CAD build for the part. Positions are in the model's coordinates, mm. A direction names the side the tool comes from. Round coordinates to 2 decimals unless told otherwise and drop trailing zeros. Write each loop counter-clockwise with the first axis right and the second up, starting at its lowest first coordinate (ties: lowest second). Pieces come first, ordered by that corner, then holes. Notation, with made-up numbers: (-11.5, 59.5) - (9.5, 59.5) arc R23 ccw to (9.5, 92.5) - close; hole circle Ø8 at (36, 61). An arc over 180 degrees is marked (long way). Use one line per item in the form item = value. Start each with the question number.
Item 1: Band-saw the part on B-B, the plane x = -9.5. List the corners of the cut face in (y, z).
Item 2: Band-saw the part on A-A, the plane z = -8.5. List the corners of the cut face in (x, y).
Item 3: Drill centre lines: L1, parallel to Y at x = 13, z = -8.25; L2, parallel to Z at x = -21, y = 28. Where is each one in solid material? Low to high.
Item 4: Tool access for faces 4 (the cylindrical face through (-32.723, 31.485, -2.909)), 5 (the flat face through (-30.25, 0, -6)), 6 (the cylindrical face through (-37.62, -0.475, -0.396)), 7 (the cylindrical face through (-32.723, -31.485, -2.909)), 8 (the flat face through (-1, -33.95, -5)): list every direction of +Z, -Z, +X, -X, +Y, -Y with a clear straight run to the whole face (end or side of a thin tool).
Item 5: Pull direction Y, two halves, no side cores. Call faces 1 (the flat face through (30.25, 0, -6)), 2 (the flat face through (-1, 33.95, -5)), 3 (the flat face through (-35.23, 0.48, -5.72)): +Y half, -Y half, draft (parallel to the pull), parting line (faces both ways), or undercut.
Item 6: Band-saw the part on C-C, the plane y = -4. List the corners of the cut face in (x, z), and give its area (3 significant figures).
Item 7: Pin check, flat tips, straight feed: pin 1 (10 mm diameter, centred on x = 12.5, y = -5, fed in from +Z); pin 2 (4 mm diameter, centred on x = -24, y = -6, fed in from -Z); pin 3 (1.2 mm diameter, centred on x = -33.63, z = -3.38, fed in from +Y); pin 4 (1.2 mm diameter, centred on x = 33.63, z = -3.38, fed in from -Y). Stop position of each tip, or through.
from build123d import *

# Parameters (mm, degrees)
SKETCH_1_W            = 81.9
SKETCH_1_H            = 67.9
EXTRUDE_1_DEPTH       = 10
SKETCH_2_W            = 60.5
SKETCH_2_H            = 60.5
CUT_EXTRUDE_1_DEPTH   = 8.5
CUT_EXTRUDE_4_REACH   = 91.242
M2_5X0_451_AT_2_COUNT = 2
M2_5X0_451_AT_2_PITCH = 67.264213562
CUT_EXTRUDE_5_REACH   = 81.921


with BuildPart() as part:
    # Эскиз1 → Бобышка-Вытянуть1 (new body)
    with BuildSketch(Plane.XY):
        Rectangle(SKETCH_1_W, SKETCH_1_H)
    extrude(amount=-EXTRUDE_1_DEPTH)

    # Эскиз2 → Вырез-Вытянуть1 (cut)
    with BuildSketch(Plane(origin=(0, 0, -10), x_dir=(-1, 0, 0), z_dir=(0, 0, -1))):
        Rectangle(SKETCH_2_W, SKETCH_2_H)
    extrude(amount=-CUT_EXTRUDE_1_DEPTH, mode=Mode.SUBTRACT)

    # Эскиз4 → Вырез-Вытянуть4 (cut, up to next)
    with BuildSketch(Plane(origin=(0, -33.95, -40.95), x_dir=(1, 0, 0), z_dir=(0, 1, 0)), mode=Mode.PRIVATE) as cut_extrude_4_sk1:
        with BuildLine():
            Line((39.383021279, -39.383021279), (40.95, -40.95))
            Line((40.95, -40.95), (35.6, -40.95))
            ThreePointArc((35.6, -40.95), (37.647356363, -40.542755499), (39.383021279, -39.383021279))
        make_face()
    cut_extrude_4_tool1 = extrude(cut_extrude_4_sk1.sketch, amount=CUT_EXTRUDE_4_REACH, mode=Mode.PRIVATE) & part.part
    # Эскиз4 → Вырез-Вытянуть4 (cut, up to next)
    with BuildSketch(Plane(origin=(0, -33.95, -40.95), x_dir=(1, 0, 0), z_dir=(0, 1, 0)), mode=Mode.PRIVATE) as cut_extrude_4_sk2:
        with BuildLine():
            Line((-40.95, -40.95), (-35.6, -40.95))
            ThreePointArc((-35.6, -40.95), (-37.647356363, -40.542755499), (-39.383021279, -39.383021279))
            Line((-39.383021279, -39.383021279), (-40.95, -40.95))
        make_face()
    cut_extrude_4_tool2 = extrude(cut_extrude_4_sk2.sketch, amount=CUT_EXTRUDE_4_REACH, mode=Mode.PRIVATE) & part.part
    add(cut_extrude_4_tool1.solids().sort_by_distance((39.042099, -33.95, -0.482136))[0], mode=Mode.SUBTRACT)
    add(cut_extrude_4_tool2.solids().sort_by_distance((-39.042099, -33.95, -0.482136))[0], mode=Mode.SUBTRACT)

    # Эскиз8 → Отверстие обработанное метчиком M2.5x0.451 (revolve, cut)
    with BuildSketch(Plane(origin=(33.632106781, 33.95, -3.382106781), x_dir=(0, 0, 1), z_dir=(1, 0, 0))):
        Polygon((0, 0), (0, 5.615882135), (1.025, 5), (1.025, 0), align=None)
    m2_5x0_451 = revolve(axis=Axis((33.632106781, 40.3, -3.382106781), (0, -1, 0)), mode=Mode.SUBTRACT)

    # Отверстие обработанное метчиком M2.5x0.451 at 2: Отверстие обработанное метчиком M2.5x0.451 ×2
    with Locations(*[(-i * M2_5X0_451_AT_2_PITCH, 0, 0) for i in range(1, M2_5X0_451_AT_2_COUNT)]):
        add(m2_5x0_451, mode=Mode.SUBTRACT)

    # Зеркальное отражение1: Отверстие обработанное метчиком M2.5x0.451 across plane
    add(m2_5x0_451.mirror(Plane.ZX), mode=Mode.SUBTRACT)

    # Зеркальное отражение1 copy 1 sketch → Зеркальное отражение1 copy 1 (revolve, cut)
    with BuildSketch(Plane(origin=(-33.632106781, -33.95, -3.382106781), x_dir=(0, 0, 1), z_dir=(1, 0, 0))):
        Polygon((0, 0), (0, -5.615882135), (1.025, -5), (1.025, 0), align=None)
    revolve(axis=Axis((-33.632106781, -40.3, -3.382106781), (0, -1, 0)), mode=Mode.SUBTRACT)

    # Эскиз3 → Вырез-Вытянуть5 (cut, up to next)
    with BuildSketch(Plane(origin=(0, 33.95, 0), x_dir=(1, 0, 0), z_dir=(0, 1, 0)), mode=Mode.PRIVATE) as cut_extrude_5_sk1:
        Polygon((30.95, 10), (40.95, 0), (40.95, 10), align=None)
    cut_extrude_5_tool1 = extrude(cut_extrude_5_sk1.sketch, amount=-CUT_EXTRUDE_5_REACH, mode=Mode.PRIVATE) & part.part
    # Эскиз3 → Вырез-Вытянуть5 (cut, up to next)
    with BuildSketch(Plane(origin=(0, 33.95, 0), x_dir=(1, 0, 0), z_dir=(0, 1, 0)), mode=Mode.PRIVATE) as cut_extrude_5_sk2:
        Polygon((-30.95, 10), (-40.95, 10), (-40.95, 0), align=None)
    cut_extrude_5_tool2 = extrude(cut_extrude_5_sk2.sketch, amount=-CUT_EXTRUDE_5_REACH, mode=Mode.PRIVATE) & part.part
    add(cut_extrude_5_tool1.solids().sort_by_distance((37.616667, 33.95, -6.666667))[0], mode=Mode.SUBTRACT)
    add(cut_extrude_5_tool2.solids().sort_by_distance((-37.616667, 33.95, -6.666667))[0], mode=Mode.SUBTRACT)


solid = part.part
Determined:
q1.outline = (-33.95, -10) - (-30.25, -10) - (-30.25, -1.5) - (30.25, -1.5) - (30.25, -10) - (33.95, -10) - (33.95, 0) - (-33.95, 0) - close
q2.outline = (-32.45, -33.95) - (32.45, -33.95) - (32.45, 33.95) - (-32.45, 33.95) - close; hole (-30.25, -30.25) - (30.25, -30.25) - (30.25, 30.25) - (-30.25, 30.25) - close
q3.L1 = -33.95 to -30.25, 30.25 to 33.95
q3.L2 = -1.5 to 0
q4.face_4 = +Y
q4.face_5 = -Z
q4.face_6 = +Z, -X, +Y, -Y
q4.face_7 = -Y
q4.face_8 = +Z, -Z, +X, -X, -Y
q5.face_1 = undercut
q5.face_2 = +Y half
q5.face_3 = draft
q6.outline = (-39.38, -1.57) - (-30.95, -10) - (-30.25, -10) - (-30.25, -1.5) - (30.25, -1.5) - (30.25, -10) - (30.95, -10) - (39.38, -1.57) arc R5.35 ccw to (35.6, 0) - (-35.6, 0) arc R5.35 ccw to start
q6.area = 199 mm²
q7.pin_1 = 0
q7.pin_2 = -1.5
q7.pin_3 = 28.7
q7.pin_4 = -28.7
